Check sheet for the drawn part. Datum: minimum x, y, z corner. Units: mm. Give positions to 0.01 mm unless a question says otherwise; leave off trailing zeros. Order: outer loops, then holes, each group sorted by start corner. A loop starts at its lowest first (then second) coordinate and runs counter-clockwise, first axis right, second up. Notation, with made-up numbers: M 7.25,66.25 L 52.25,66.25 A16 ccw 52.25,78.25 Z; hole C -27,-36.75 d11. An arc over 180 degrees is marked long. One line per question, with ' | ' between items. Start each with the question number.
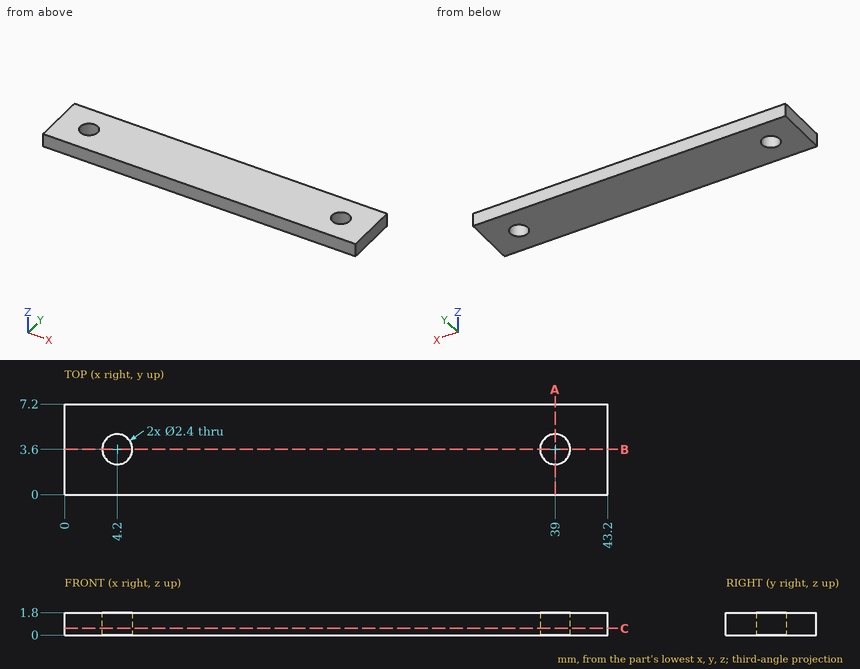
Item 1: Section check B-B, the plane y = 3.6. Record the cut outline in (x, z).
Item 2: Section check A-A, the plane x = 39. Record the cut outline in (y, z), then the cut area to 3 significant figures.
Item 3: Section check C-C, the plane z = 0.55. Record the cut outline in (x, y).
Item 4: Scan lines: probe 1 along X at (y, z) = (3.5, 0.4); probe 2 along Y at (x, z) = (4.2, 1.2); probe 3 along Y at (x, z) = (38.5, 1). Record each from-to range of solid material in increasing order. Write a range as [from, to].
Reported:
1) outline: M 0,0 L 3,0 L 3,1.8 L 0,1.8 Z; M 5.4,0 L 37.8,0 L 37.8,1.8 L 5.4,1.8 Z; M 40.2,0 L 43.2,0 L 43.2,1.8 L 40.2,1.8 Z
2) outline: M 0,0 L 2.4,0 L 2.4,1.8 L 0,1.8 Z; M 4.8,0 L 7.2,0 L 7.2,1.8 L 4.8,1.8 Z | area: 8.64 mm^2
3) outline: M 0,0 L 43.2,0 L 43.2,7.2 L 0,7.2 Z; hole C 4.2,3.6 d2.4; hole C 39,3.6 d2.4
4) probe 1: x = [0, 3], [5.4, 37.8], [40.2, 43.2] | probe 2: y = [0, 2.4], [4.8, 7.2] | probe 3: y = [0, 2.51], [4.69, 7.2]
